from build123d import *

# Parameters (mm, degrees)
F2_R      = 20
F0_R      = 22.5
F4_T      = -1
F5_R      = 20
F7_R      = 10
F9_R      = 10.2
F10_DEPTH = 25


with BuildPart() as f3:
    # F2 (on offset) → F3 section 0
    with BuildSketch(Plane.XY.offset(10)):
        Circle(F2_R)
    # F0 (on Top) → F3 section 1
    with BuildSketch(Plane.XY):
        Circle(F0_R)
    loft()

    # F4
    f4_openings = [f3.faces().sort_by_distance(p)[0] for p in [
        (0, 0, 0),
    ]]
    offset(amount=F4_T, openings=f4_openings, kind=Kind.INTERSECTION)

    # F5 (on face) → F8 section 0
    with BuildSketch(Plane.XY.offset(10)):
        Circle(F5_R)
    # F7 (on offset) → F8 section 1
    with BuildSketch(Plane.XY.offset(40)):
        Circle(F7_R)
    loft()

    # F9 (on face) → F10 (cut)
    with BuildSketch(Plane(origin=(0, 0, 9), x_dir=(1, 0, 0), z_dir=(0, 0, -1))):
        Circle(F9_R)
    extrude(amount=-F10_DEPTH, mode=Mode.SUBTRACT)

    # F11 (on Front) → F12 (revolve)
    with BuildSketch(Plane.XZ):
        with BuildLine():
            Line((0, 68.8017484976), (0, 40))
            Line((0, 40), (10, 40))
            ThreePointArc((10, 40), (15.2441850924, 57.9576670224), (0, 68.8017484976))
        make_face()
    revolve(axis=Axis((0, 0, 56.8208959699), (0, 0, -1)))


solid = f3.part
The listing builds one solid part. Answer for the finished solid, in the listing's coordinates (mm). A direction names the side the tool comes from. Give positions to 0.01 mm unless a question says otherwise; leave off trailing zeros. Write each loop counter-clockwise with the first axis right and the second up, starting at its lowest first coordinate (ties: lowest second). Pieces come first, ordered by that corner, then holes.
Item 1: Which of the six approach directions +Z, -Z, +X, -X, +Y, -Y give full straight-line access (tool end or side, diameter ignored) to faces 1 (the conical face through (19.23, 6.05, 9.37)), 2 (the cylindrical face through (4.707, 9.049, 21.325))?
Item 2: Section A-A, the plane z = 31 is taken. Write down the section's boundary in (x, y).
Item 3: Determine the mould class of faces 3 (the flat face through (0, 0, 34)), 4 (the conical face through (6.38, -12.26, 28.54)), 5 (the flat face through (12, -18, 0)), 6 (the flat face through (8, -8, 9)) for opening direction Y: released by +Y, released by -Y, zero draft, split by the parting line, or undercut.
Item 4: Find the intervals of material crossed by line 1 along Z through (x, y) = (8, -9.5); line 2 along Y through (x, z) = (0, 28.5); line 3 along Y through (x, z) = (0, 14.75), in increasing order.
Item 5: Section D-D, the plane z = 45 is taken. Write down the section's boundary in (x, y), plus the area to 3 significant figures.
Item 6: Section C-C, the plane z = 63.5 is taken. Write down the section's boundary in (x, y).
Item 7: Flat-ended cylindrical pins translate along their axes: P1, Ø5, axis at y = 5.5, z = 12, coming from the +X side; P2, Ø1.5, axis at x = -12.5, z = 61, coming from the -Y side; P3, Ø1.5, axis at y = 11, z = 28, coming from the -X side. Find the tip coordinate at first contact, or state that the pin passes through.
Item 8: Section B-B, the plane x = 0 is taken. Write down the section's boundary in (y, z).
Completed:
1. face 1: +Z
1. face 2: -Z
2. outline: circle Ø26 at (0, 0); hole circle Ø20.4 at (0, 0)
3. face 3: undercut
3. face 4: split by the parting line
3. face 5: zero draft
3. face 6: undercut
4. line 1: z = 9 to 32.74, 42.36 to 62.97
4. line 2: y = -13.83 to -10.2, 10.2 to 13.83
4. line 3: y = -18.42 to -10.2, 10.2 to 18.42
5. outline: circle Ø28.4 at (0, 0)
5. area: 633 mm2
6. outline: circle Ø23.92 at (0, 0)
7. P1: stops at x = 19.6
7. P2: stops at y = -7.53
7. P3: stops at x = -9.62
8. outline: (-22.5, 0) - (-21.47, 0) - (-19.22, 9) - (-10.2, 9) - (-10.2, 34) - (10.2, 34) - (10.2, 9) - (19.22, 9) - (21.47, 0) - (22.5, 0) - (20, 10) - (10, 40) arc R16.14 ccw (long way) to (-10, 40) - (-20, 10) - close
